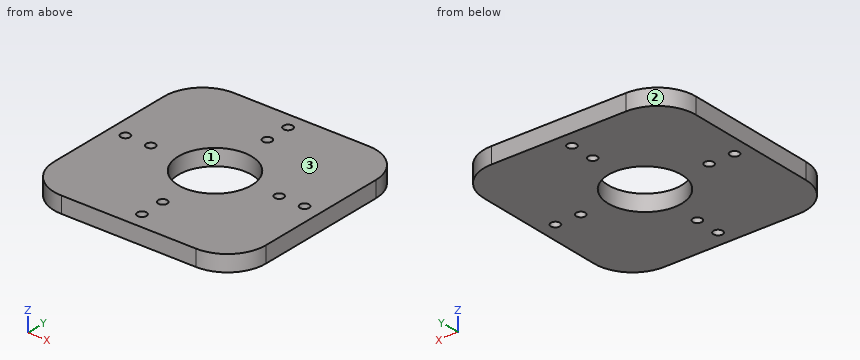
from build123d import *

# Parameters (mm, degrees)
F0_W     = 82.55
F0_H     = 82.55
F0_R     = 1.778
F0_R_2   = 14.2875
F1_DEPTH = 6.35
F2_R     = 15


# Not quite as in the source:
# - a length typed as a fraction of an inch, garbled in the dataset ("3 / 203.2 mm" for 3/8 in), is restored


with BuildPart() as f1:
    # F0 (on Top) → F1 (new body)
    with BuildSketch(Plane.XY):
        Rectangle(F0_W, F0_H)
        with Locations((0, -34.925)):
            Circle(F0_R, mode=Mode.SUBTRACT)
        with Locations((0, -25)):
            Circle(F0_R, mode=Mode.SUBTRACT)
        with Locations((-34.925, 0)):
            Circle(F0_R, mode=Mode.SUBTRACT)
        with Locations((-25, 0)):
            Circle(F0_R, mode=Mode.SUBTRACT)
        Circle(F0_R_2, mode=Mode.SUBTRACT)
        with Locations((25, 0)):
            Circle(F0_R, mode=Mode.SUBTRACT)
        with Locations((34.925, 0)):
            Circle(F0_R, mode=Mode.SUBTRACT)
        with Locations((0, 25)):
            Circle(F0_R, mode=Mode.SUBTRACT)
        with Locations((0, 34.925)):
            Circle(F0_R, mode=Mode.SUBTRACT)
    extrude(amount=F1_DEPTH)

    # F2
    f2_edges = [f1.edges().sort_by_distance(p)[0] for p in [
        (-41.275, 41.275, 3.175),
        (-41.275, -41.275, 3.175),
        (41.275, 41.275, 3.175),
        (41.275, -41.275, 3.175),
    ]]
    fillet(f2_edges, radius=F2_R)


solid = f1.part
Build history of the part. All positions in model axes, mm. Face numbers are marked on the shaded views. Give positions to 0.01 mm unless a question says otherwise; leave off trailing zeros. Order: outer loops, then holes, each group sorted by start corner. A loop starts at its lowest first (then second) coordinate and runs counter-clockwise, first axis right, second up. Notation, with made-up numbers: M -10,-18 L 39,-18 A32 cw 39,21 Z; hole C 45.25,37.25 d10. An arc over 180 degrees is marked long. Use one line per item in the form item = value.
Q1. Pin check, flat tip, straight feed: P1, Ø3, axis at x = 0, y = -34.925, coming from the -Z side. Stop position of the tip, or through.
Conclusion:
P1 = through
Q2. Pull direction X, two halves, no side cores. Call the marked faces 1, 2 and 3: released by +X, released by -X, zero draft, split by the parting line, or undercut.
Conclusion:
face_1 = undercut
face_2 = released by -X
face_3 = zero draft
Q3. Wall check: probe 1 along Y at (x, z) = (0, 4.75) (1 decimal); probe 2 along X at (y, z) = (1, 5) (3 decimals); probe 3 along Y at (x, z) = (-0.5, 5.5) (3 decimals). Give the ranges that are in metal, low to high.
Conclusion:
probe_1 = -41.3 to -36.7, -33.1 to -26.8, -23.2 to -14.3, 14.3 to 23.2, 26.8 to 33.1, 36.7 to 41.3
probe_2 = -41.275 to -36.395, -33.455 to -26.47, -23.53 to -14.252, 14.252 to 23.53, 26.47 to 33.455, 36.395 to 41.275
probe_3 = -41.275 to -36.631, -33.219 to -26.706, -23.294 to -14.279, 14.279 to 23.294, 26.706 to 33.219, 36.631 to 41.275
Q4. Slice it at A-A, the plane x = -25. Write the cut outline in (y, z) (3 decimals).
Conclusion:
outline = M -41.275,0 L -1.778,0 L -1.778,6.35 L -41.275,6.35 Z; M 1.778,0 L 41.275,0 L 41.275,6.35 L 1.778,6.35 Z
Q5. Slice it at C-C, the plane y = 0. State how many separate pieces and enclosed holes the cut face has, and give its area (3 significant figures).
Conclusion:
separate_pieces = 6
enclosed_holes = 0
area = 252 mm2
